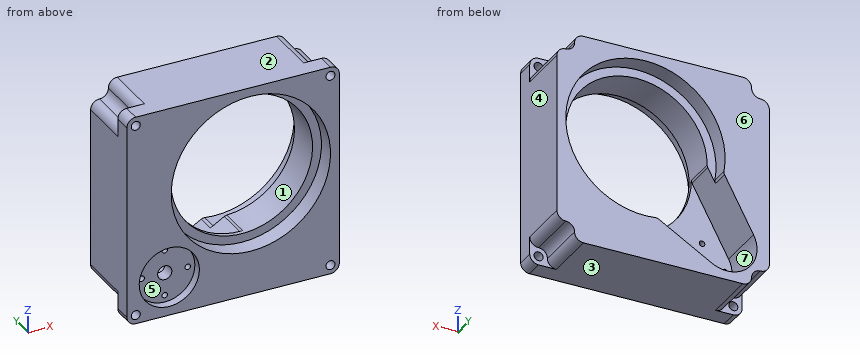
```python
from build123d import *

# Parameters (mm, degrees)
SKETCH1_W           = 120
SKETCH1_H           = 120
BOSS_EXTRUDE1_DEPTH = 40
SKETCH2_R           = 40
CUT_EXTRUDE1_DEPTH  = 94.808315196
SKETCH3_R           = 45
CUT_EXTRUDE2_DEPTH  = 10
CUT_EXTRUDE3_START  = -10
SKETCH4_R           = 45
CUT_EXTRUDE3_DEPTH  = 10
SKETCH11_W          = 10
SKETCH11_H          = 10
CUT_EXTRUDE8_DEPTH  = 30
SKETCH7_R           = 17
CUT_EXTRUDE5_DEPTH  = 27.5
CUT_EXTRUDE10_START = -5
SKETCH13_R          = 17
CUT_EXTRUDE10_DEPTH = 5
SKETCH14_R          = 4
SKETCH14_R_2        = 1.55
CUT_EXTRUDE11_DEPTH = 90.197813875
CUT_EXTRUDE7_REACH  = 95.808
SKETCH12_R          = 2.55
CUT_EXTRUDE9_DEPTH  = 91
FILLET1_R           = 5
FILLET2_R           = 5
FILLET3_R           = 3


with BuildPart() as part:
    # Sketch1 → Boss-Extrude1 (new body)
    with BuildSketch(Plane(origin=(0, 0, 0), x_dir=(1, 0, 0), z_dir=(0, 1, 0))):
        Rectangle(SKETCH1_W, SKETCH1_H)
    extrude(amount=BOSS_EXTRUDE1_DEPTH)

    # Sketch2 → Cut-Extrude1 (cut, through all)
    with BuildSketch(Plane(origin=(0, 40, 0), x_dir=(1, 0, 0), z_dir=(0, 1, 0))):
        with Locations(Location((10, -10, 0), (0, 0, 270))):
            Circle(SKETCH2_R)
    extrude(amount=-CUT_EXTRUDE1_DEPTH, mode=Mode.SUBTRACT)

    # Sketch3 → Cut-Extrude2 (cut)
    with BuildSketch(Plane(origin=(0, 40, 0), x_dir=(1, 0, 0), z_dir=(0, 1, 0))):
        with Locations(Location((10, -10, 0), (0, 0, 270))):
            Circle(SKETCH3_R)
    extrude(amount=-CUT_EXTRUDE2_DEPTH, mode=Mode.SUBTRACT)

    # Sketch4 → Cut-Extrude3 (cut)
    with BuildSketch(Plane.XZ.offset(CUT_EXTRUDE3_START)):
        with Locations(Location((10, 10, 0), (0, 0, 90))):
            Circle(SKETCH4_R)
    extrude(amount=CUT_EXTRUDE3_DEPTH, mode=Mode.SUBTRACT)

    # Sketch11 → Cut-Extrude8 (cut)
    with BuildSketch(Plane(origin=(0, 40, 0), x_dir=(1, 0, 0), z_dir=(0, 1, 0))):
        with Locations((-55, 55)):
            Rectangle(SKETCH11_W, SKETCH11_H)
        with Locations((55, 55)):
            Rectangle(SKETCH11_W, SKETCH11_H)
        with Locations((55, -55)):
            Rectangle(SKETCH11_W, SKETCH11_H)
        with Locations((-55, -55)):
            Rectangle(SKETCH11_W, SKETCH11_H)
    extrude(amount=-CUT_EXTRUDE8_DEPTH, mode=Mode.SUBTRACT)

    # Sketch7 → Cut-Extrude5 (cut)
    with BuildSketch(Plane(origin=(0, 40, 0), x_dir=(1, 0, 0), z_dir=(0, 1, 0))):
        with Locations(Location((-36.059780402, 37.96609875, 0), (0, 0, 270))):
            Circle(SKETCH7_R)
    extrude(amount=-CUT_EXTRUDE5_DEPTH, mode=Mode.SUBTRACT)

    # Sketch13 → Cut-Extrude10 (cut)
    with BuildSketch(Plane.XZ.offset(CUT_EXTRUDE10_START)):
        with Locations(Location((-36.059780402, -37.96609875, 0), (0, 0, 90))):
            Circle(SKETCH13_R)
    extrude(amount=CUT_EXTRUDE10_DEPTH, mode=Mode.SUBTRACT)

    # Sketch14 → Cut-Extrude11 (cut, through all)
    with BuildSketch(Plane(origin=(0, 12.5, 0), x_dir=(1, 0, 0), z_dir=(0, 1, 0))):
        with Locations(Location((-36.059780402, 37.96609875, 0), (0, 0, 270))):
            Circle(SKETCH14_R)
        with Locations(Location((-36.059780402, 50.96609875, 0), (0, 0, 270))):
            Circle(SKETCH14_R_2)
        with Locations(Location((-23.059780402, 37.96609875, 0), (0, 0, 270))):
            Circle(SKETCH14_R_2)
        with Locations(Location((-36.059780402, 24.96609875, 0), (0, 0, 270))):
            Circle(SKETCH14_R_2)
        with Locations(Location((-49.059780402, 37.96609875, 0), (0, 0, 270))):
            Circle(SKETCH14_R_2)
    extrude(amount=-CUT_EXTRUDE11_DEPTH, mode=Mode.SUBTRACT)

    # Cut-Extrude7: up to this face of the body (flat: up to its plane)
    cut_extrude7_end = Plane(part.part.faces().sort_by_distance((-36.059780402, 12.5, -54.485266139))[0])
    # Sketch10 → Cut-Extrude7 (cut, up to the picked face)
    with BuildSketch(Plane(origin=(0, 40, 0), x_dir=(1, 0, 0), z_dir=(0, 1, 0)), mode=Mode.PRIVATE) as cut_extrude7_sk1:
        with BuildLine():
            Line((-27.442638837, 52.620274648), (27.741173812, 20.170362142))
            ThreePointArc((27.741173812, 20.170362142), (34.241989685, -35.245315132), (-20.864656949, -26.503725379))
            Line((-20.864656949, -26.503725379), (-51.051185206, 29.950003566))
            ThreePointArc((-51.051185206, 29.950003566), (-47.834461107, 50.228108957), (-27.442638837, 52.620274648))
        make_face()
    cut_extrude7_tool1 = split(extrude(cut_extrude7_sk1.sketch, amount=-CUT_EXTRUDE7_REACH, mode=Mode.PRIVATE), bisect_by=cut_extrude7_end, keep=Keep.BOTH, mode=Mode.PRIVATE)
    add(cut_extrude7_tool1.solids().sort_by(Axis((-2.85152, 40, -3.383418), (0, -1, 0)))[0], mode=Mode.SUBTRACT)

    # Sketch12 → Cut-Extrude9 (cut, through all)
    with BuildSketch(Plane(origin=(0, 10, 0), x_dir=(1, 0, 0), z_dir=(0, 1, 0))):
        with Locations(Location((-55, 55, 0), (0, 0, 270))):
            Circle(SKETCH12_R)
        with Locations(Location((55, 55, 0), (0, 0, 270))):
            Circle(SKETCH12_R)
        with Locations(Location((55, -55, 0), (0, 0, 270))):
            Circle(SKETCH12_R)
        with Locations(Location((-55, -55, 0), (0, 0, 270))):
            Circle(SKETCH12_R)
    extrude(amount=-CUT_EXTRUDE9_DEPTH, mode=Mode.SUBTRACT)

    # Fillet1
    fillet1_edges = [part.edges().sort_by_distance(p)[0] for p in [
        (-60, 5, -60),
        (-50, 25, -50),
        (60, 5, -60),
        (50, 25, -50),
        (60, 5, 60),
        (50, 25, 50),
        (-60, 5, 60),
        (-50, 25, 50),
    ]]
    fillet(fillet1_edges, radius=FILLET1_R)

    # Fillet2
    fillet2_edges = [part.edges().sort_by_distance(p)[0] for p in [
        (50, 25, -60),
        (60, 25, -50),
        (60, 25, 50),
        (-50, 25, 60),
        (-60, 25, 50),
        (-50, 25, -60),
        (-60, 25, -50),
        (50, 25, 60),
    ]]
    fillet(fillet2_edges, radius=FILLET2_R - 0.0001)  # a hair under: the kernel refuses the full size

    # Fillet3
    fillet3_edges = [part.edges().sort_by_distance(p)[0] for p in [
        (-29.99589317, 21.25, 9.426825043),
        (-34.201681099, 35, 1.561315976),
        (11.048415222, 21.25, -29.986257958),
        (3.359839341, 35, -34.507395637),
    ]]
    fillet(fillet3_edges, radius=FILLET3_R)


solid = part.part
```
Here's how the part is built. I have some questions about the finished solid (model axes, mm). Face numbers are marked on the shaded views. A direction names the side the tool comes from. Give positions to 0.01 mm unless a question says otherwise; leave off trailing zeros. Write each loop counter-clockwise with the first axis right and the second up, starting at its lowest first coordinate (ties: lowest second). Pieces come first, ordered by that corner, then holes. Notation, with made-up numbers: M -39.5,18.25 L -24.5,18.25 A19 ccw -24.5,37.25 Z; hole C -23,49 d3. An arc over 180 degrees is marked long. Put each result on its own line as item: value. Start each with the question number.
Item 1: If we section it at B-B, the plane x = -12: Write out the boundary of the cut face in (y, z).
Item 2: If we section it at C-C, the plane z = -6.5: Write out the boundary of the cut face in (x, y), then the cut area to 3 significant figures.
Item 3: Thinking about a two-plate mould opening in Z: for the marked faces 1, 2, 3 and 4, which applies, +Z half, -Z half, draft (parallel to the pull), parting line (faces both ways), or undercut?
Item 4: On a 3-axis mill with a long thin cutter (end or side, diameter ignored), from which of +Z, -Z, +X, -X, +Y, -Y can I reach the whole of each face in a straight line? I mean the marked faces 5, 6 and 7. Say none if no direction works.
Item 5: If we section it at D-D, the plane y = 6.5: Count the separate pieces of the cut face and the enclosed holes in it, then the cut area to 3 significant figures.
Item 6: I need wall thicknesses on L1, parallel to X at y = 7.5, z = -55; L2, parallel to X at y = 23, z = 11.5; L3, parallel to Z at x = -26, y = 29. Which ranges of each line are inside material? Lowest first, please. Write a range as from..to.
Item 7: Will this pin go through, and if not, where does the flat tip stop? pin 1 (4 mm diameter, centred on x = -36.06, z = -50.97, fed in from +Y).
Values:
1. outline: M 0,-60 L 40,-60 L 40,-43.54 L 12.5,-43.54 L 12.5,-23.41 L 10,-23.41 L 10,-29.26 L 0,-29.26 Z; M 0,49.26 L 10,49.26 L 10,43.41 L 30,43.41 L 30,49.26 L 40,49.26 L 40,60 L 0,60 Z
2. outline: M -60,0 L -31.87,0 L -31.87,10 L -26.44,10 L -26.44,12.5 L -38.51,12.5 L -38.51,40 L -60,40 Z; M 46.44,10 L 51.87,10 L 51.87,0 L 60,0 L 60,40 L 51.87,40 L 51.87,30 L 46.44,30 Z
2. area: 1,390 mm²
3. face 1: undercut
3. face 2: +Z half
3. face 3: -Z half
3. face 4: draft
4. face 5: -Y
4. face 6: +Z, -Z, +X, -X, +Y
4. face 7: +Y
5. separate pieces: 1
5. enclosed holes: 10
5. area: 7,850 mm²
6. L1: -60..-57.55, -52.45..52.45, 57.55..60
6. L2: -60..-29.97, 49.97..60
6. L3: -60..-51.77, 27.44..60
7. pin 1: y = 12.5
